```python
from build123d import *

# Parameters (mm, degrees)
SWEEP1_PROFILE_R = 33.528
SWEEP2_PROFILE_R = 6.35
SWEEP3_PROFILE_R = 6.35


with BuildPart() as part:
    # Sweep1: sweep along a path in Sketch1
    with BuildLine(Plane.XY) as sweep1_path:
        Line((-48.641, 0), (48.641, 0))
    # Sweep1 profile (on start of the path) → Sweep1 (sweep)
    with BuildSketch(Plane.YZ.offset(-48.641)):
        Circle(SWEEP1_PROFILE_R)
    sweep(path=sweep1_path.line)

    # Sweep2: sweep along a path in Sketch11
    with BuildLine(Plane.XY) as sweep2_path:
        Line((48.641, 0), (67.183, 0))
    # Sweep2 profile (on start of the path) → Sweep2 (sweep)
    with BuildSketch(Plane.YZ.offset(48.641)):
        Circle(SWEEP2_PROFILE_R)
    sweep(path=sweep2_path.line)

    # Sweep3: sweep along a path in Sketch30
    with BuildLine(Plane.XY) as sweep3_path:
        Line((-48.641, 0), (-67.183, 0))
    # Sweep3 profile (on start of the path) → Sweep3 (sweep)
    with BuildSketch(Plane(origin=(-48.641, 0, 0), x_dir=(0, -1, 0), z_dir=(-1, 0, 0))):
        Circle(SWEEP3_PROFILE_R)
    sweep(path=sweep3_path.line)


solid = part.part
```
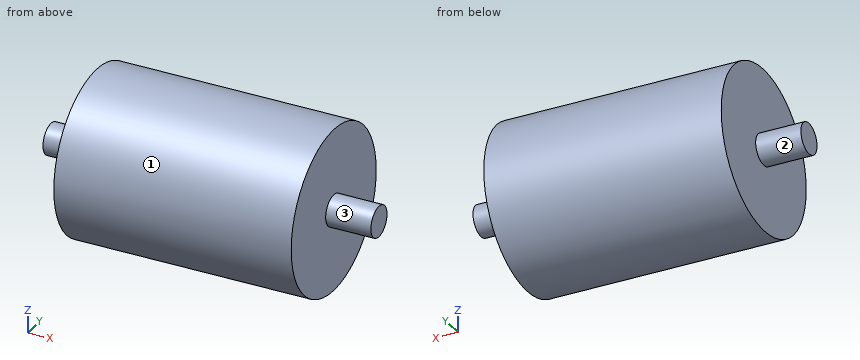
Work out the finished part from the listing and answer in its coordinate system (mm). Face numbers are marked on the shaded views. A direction names the side the tool comes from. Give positions to 0.01 mm unless a question says otherwise; leave off trailing zeros. Write each loop counter-clockwise with the first axis right and the second up, starting at its lowest first coordinate (ties: lowest second). Pieces come first, ordered by that corner, then holes.
(1) The part is cut by section A-A on z = 0. Write down the section's boundary in (x, y).
Final values:
outline: (-67.18, -6.35) - (-48.64, -6.35) - (-48.64, -33.53) - (48.64, -33.53) - (48.64, -6.35) - (67.18, -6.35) - (67.18, 6.35) - (48.64, 6.35) - (48.64, 33.53) - (-48.64, 33.53) - (-48.64, 6.35) - (-67.18, 6.35) - close
(2) The part is cut by section D-D on x = -53. Write down the section's boundary in (y, z), plus the area to 3 significant figures.
Final values:
outline: circle Ø12.7 at (0, 0)
area: 127 mm2
(3) Straight lines are drawn through the part: line 1 (X direction, y = 16, z = 20.5); line 2 (Z direction, x = -29.5, y = 1); line 3 (Z direction, x = -10, y = -23.5). For each, find the intervals that lie inside material, in ascending order.
Final values:
line 1: x = -48.64 to 48.64
line 2: z = -33.51 to 33.51
line 3: z = -23.91 to 23.91
(4) The part is cut by section C-C on x = 3.5. Write down the section's boundary in (y, z), plus the area to 3 significant figures.
Final values:
outline: circle Ø67.06 at (0, 0)
area: 3,530 mm2
(5) Which of the six approach directions +Z, -Z, +X, -X, +Y, -Y give full straight-line access (tool end or side, diameter ignored) to the marked faces 1, 2 and 3?
Final values:
face 1: +X, -X
face 2: -X
face 3: +X
(6) Flat-ended cylindrical pins translate along their axes: pin 1 Ø2 at (x, y) = (-29.5, -20.5) entering from -Z; pin 2 Ø12 at (y, z) = (18.5, 17.5) entering from +X; pin 3 Ø1 at (x, y) = (22.5, 7) entering from -Z. Find the tip coordinate at first contact, or state that the pin passes through.
Final values:
pin 1: stops at z = -27.27
pin 2: stops at x = 48.64
pin 3: stops at z = -32.89
